Here's the drawing with two shaded views (mm, measured from the low corner). I have some questions. A direction names the side the tool comes from. Round coordinates to 2 decimals unless told otherwise and drop trailing zeros. Loops run counter-clockwise (first coordinate to the right, second up) from the corner with the lowest first, then second, coordinate; pieces in that order, holes last.
(1) I want a section at A-A on x = 2. Write out the boundary of the cut face in (y, z).
(2) I want a section at C-C on y = 1.75. Write out the boundary of the cut face in (x, z).
(3) Which directions (+Z, -Z, +X, -X, +Y, -Y) give clear straight access to the entire face, cutting with the end or side of a thin tool? Please do the marked faces 1, 2 and 3.
(4) I want a section at D-D on z = 8.5. Write out the boundary of the cut face in (x, y).
(5) Thinking about a two-plate mould opening in Z: for the marked faces 4, 5, 6 and 7, which applies, released by +Z, released by -Z, zero draft, split by the parting line, or undercut?
(6) If I drill on line 1 along Z through (x, y) = (23, 1.8); line 2 along X through (y, z) = (3.5, 4.5); line 3 along Y through (x, z) = (22, 4), over which ranges is the centre line in solid material (lowest first)?
(7) I want a section at B-B on z = 5. Write out the boundary of the cut face in (x, y), plus the area to 3 significant figures.
(8) Will these pins go through, and if not, where does the flat tip stop? pin 1 Ø6 at (x, z) = (18, 3.5) entering from +Y; pin 2 Ø4 at (x, z) = (16, 2) entering from +Y; pin 3 Ø3 at (y, z) = (6, 8.5) entering from -X.
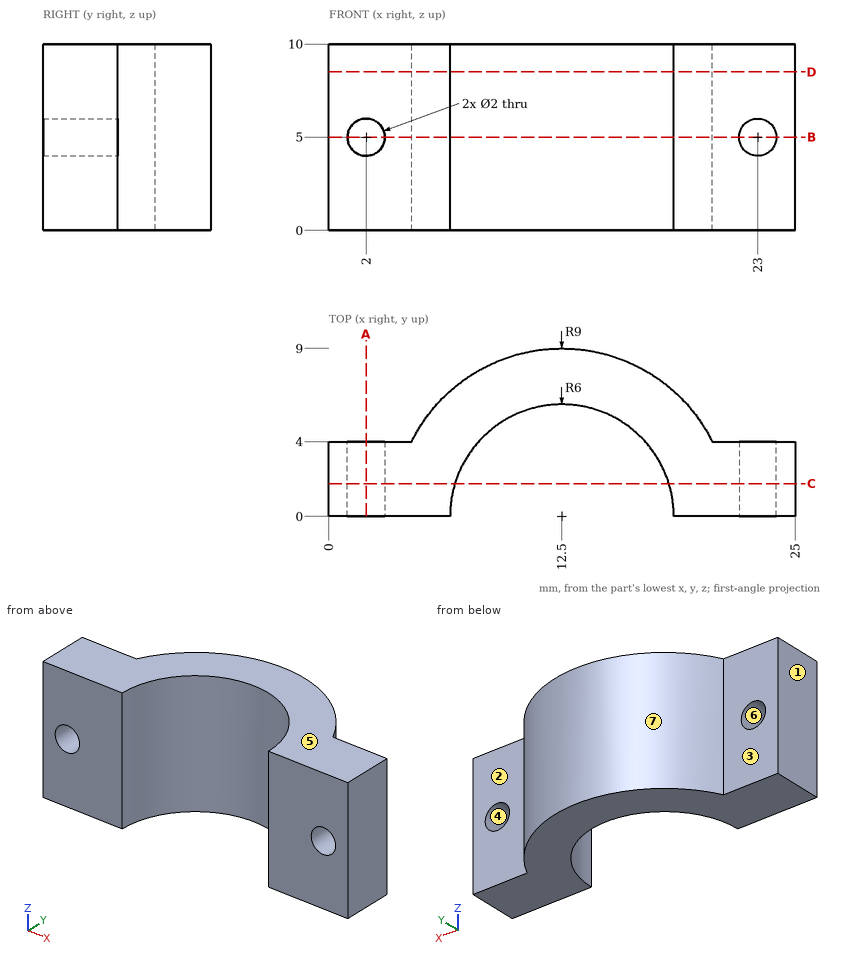
Filled sheet:
1. outline: (0, 0) - (4, 0) - (4, 4) - (0, 4) - close; (0, 6) - (4, 6) - (4, 10) - (0, 10) - close
2. outline: (0, 0) - (6.76, 0) - (6.76, 10) - (0, 10) - close; (18.24, 0) - (25, 0) - (25, 10) - (18.24, 10) - close; hole circle Ø2 at (2, 5); hole circle Ø2 at (23, 5)
3. face 1: +Z, -Z, -X, +Y, -Y
3. face 2: +Z, -Z, +X, +Y
3. face 3: +Z, -Z, -X, +Y
4. outline: (0, 0) - (6.5, 0) arc R6 cw to (18.5, 0) - (25, 0) - (25, 4) - (20.56, 4) arc R9 ccw to (4.44, 4) - (0, 4) - close
5. face 4: undercut
5. face 5: released by +Z
5. face 6: undercut
5. face 7: zero draft
6. line 1: z = 0 to 4, 6 to 10
6. line 2: x = 0 to 1.13, 2.87 to 7.63, 17.37 to 22.13, 23.87 to 25
6. line 3: y = 0 to 4
7. outline: (0, 0) - (1, 0) - (1, 4) - (0, 4) - close; (3, 0) - (6.5, 0) arc R6 cw to (18.5, 0) - (22, 0) - (22, 4) - (20.56, 4) arc R9 ccw to (4.44, 4) - (3, 4) - close; (24, 0) - (25, 0) - (25, 4) - (24, 4) - close
7. area: 85.1 mm2
8. pin 1: stops at y = 8.65
8. pin 2: stops at y = 8.87
8. pin 3: stops at x = 4.71
